Input: part model. Units: mm. Frame: model coordinates. Face numbers are marked on the shaded views. A direction names the side the tool comes from. Give positions to 0.01 mm unless a question says otherwise; leave off trailing zeros. Order: outer loops, then holes, each group sorted by start corner. A loop starts at its lowest first (then second) coordinate and runs counter-clockwise, first axis right, second up. Notation, with made-up numbers: (-27, 34.25) - (-2, 34.25) arc R27 cw to (-2, 73.25) - close; hole circle Ø8 at (-37.75, -14). An arc over 180 degrees is marked (long way). Use a Markdown table: item, result.
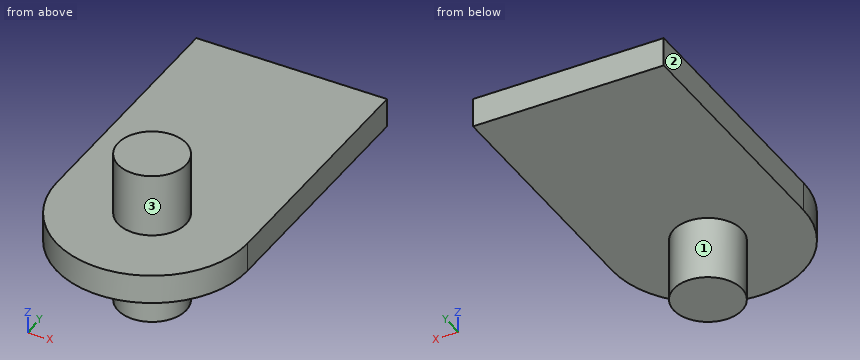
from build123d import *

# Parameters (mm, degrees)
BOSS_EXTRUDE1_DEPTH = 1.190625
SKETCH2_R           = 2.778125
BOSS_EXTRUDE2_DEPTH = 6.35


with BuildPart() as part:
    # Sketch1 → Boss-Extrude1 (new, symmetric)
    with BuildSketch(Plane.XY):
        with BuildLine():
            Line((22.568685476, 13.663463824), (22.568685476, 34.140593758))
            Line((22.568685476, 34.140593758), (7.014425609, 34.140593758))
            Line((7.014425609, 34.140593758), (7.014425609, 13.663463824))
            ThreePointArc((7.014425609, 13.663463824), (14.791555542, 5.886333891), (22.568685476, 13.663463824))
        make_face()
    extrude(amount=BOSS_EXTRUDE1_DEPTH, both=True)

    # Sketch2 → Boss-Extrude2 (add, symmetric)
    with BuildSketch(Plane.XY):
        with Locations((14.791555542, 13.663463824)):
            Circle(SKETCH2_R)
    extrude(amount=BOSS_EXTRUDE2_DEPTH, both=True)


solid = part.part
1. Material intervals for line 1 along Z through (x, y) = (20.5, 15.5); line 2 along X through (y, z) = (13.75, 2.5); line 3 along Y through (x, z) = (13, -5.5), sorted ascending.
Response:
| item | result |
|---|---|
| line 1 | z = -1.19 to 1.19 |
| line 2 | x = 12.01 to 17.57 |
| line 3 | y = 11.54 to 15.79 |
2. Section query C-C (y = 9.75). Return loops of the section in (x, z), then the cut area to 3 significant figures.
Response:
| item | result |
|---|---|
| outline | (8.07, -1.19) - (21.51, -1.19) - (21.51, 1.19) - (8.07, 1.19) - close |
| area | 32.0 mm^2 |
3. Section query B-B (x = 16.25). Return loops of the section in (y, z).
Response:
| item | result |
|---|---|
| outline | (6.02, -1.19) - (11.3, -1.19) - (11.3, -6.35) - (16.03, -6.35) - (16.03, -1.19) - (34.14, -1.19) - (34.14, 1.19) - (16.03, 1.19) - (16.03, 6.35) - (11.3, 6.35) - (11.3, 1.19) - (6.02, 1.19) - close |
4. Pin query (flat end, axial travel): pin 1 (3 mm diameter, centred on x = 19, y = 29.5, fed in from -Z); pin 2 (4.5 mm diameter, centred on x = 11.5, y = 18.5, fed in from +Z); pin 3 (4 mm diameter, centred on y = 29, z = -3, fed in from +X); pin 4 (4 mm diameter, centred on y = 9, z = 3, fed in from -X). Return the tip coordinate at first contact, or that it passes through.
Response:
| item | result |
|---|---|
| pin 1 | stops at z = -1.19 |
| pin 2 | stops at z = 1.19 |
| pin 3 | stops at x = 22.57 |
| pin 4 | stops at x = 8.01 |
5. Section query D-D (z = 0.75). Return loops of the section in (x, y), then the cut area to 3 significant figures.
Response:
| item | result |
|---|---|
| outline | (7.01, 13.66) arc R7.78 ccw to (22.57, 13.66) - (22.57, 34.14) - (7.01, 34.14) - close |
| area | 414 mm^2 |
6. Section query A-A (z = -5). Return loops of the section in (x, y), then the cut area to 3 significant figures.
Response:
| item | result |
|---|---|
| outline | circle Ø5.56 at (14.79, 13.66) |
| area | 24.2 mm^2 |
7. Set-up query: the marked faces 1, 2 and 3. Return all of +Z, -Z, +X, -X, +Y, -Y with unobstructed straight access to the full face (end or side cutting, diameter ignored); none if empty.
Response:
| item | result |
|---|---|
| face 1 | -Z |
| face 2 | +Z, -Z, -X, +Y, -Y |
| face 3 | +Z |
